The listing builds one solid part. Answer for the finished solid, in the listing's coordinates (mm). Face numbers are marked on the shaded views. A direction names the side the tool comes from. Give positions to 0.01 mm unless a question says otherwise; leave off trailing zeros. Order: outer loops, then holes, each group sorted by start corner. A loop starts at its lowest first (then second) coordinate and runs counter-clockwise, first axis right, second up. Notation, with made-up numbers: (65.25, -4) - (91.25, -4) arc R21 cw to (91.25, 7) - close; hole circle Ø8 at (-22, -11). An arc over 180 degrees is marked (long way). Use a Markdown table: item, result. Add a question column.
1) Find section A-A, the plane x = 90. Determine the outline of the cut face in (y, z).
2) For the marked faces 1 and 2, determine the directions among +Z, -Z, +X, -X, +Y, -Y from which every point of the face is accessible in a straight line to the end or side of a thin tool.
3) Straight lines are drawn through the part: line 1 (Y direction, x = -90, z = -52.4); line 2 (Z direction, x = -64, y = 19); line 3 (Y direction, x = -13, z = 21.5). For each, find the intervals that lie inside material, in ascending order.
4) Find section B-B, the plane y = 20. Determine the outline of the cut face in (x, z).
5) Flat-ended cylindrical pins translate along their axes: pin 1 (12 mm diameter, centred on x = 28, z = -39, fed in from +Y); pin 2 (12.5 mm diameter, centred on x = 2.5, y = 19, fed in from +Z). Find the tip coordinate at first contact, or state that the pin passes through.
6) Find section C-C, the plane z = 4. Determine the outline of the cut face in (x, y), plus the area to 3 significant figures.
7) Find section D-D, the plane x = -72. Determine the outline of the cut face in (y, z), plus the area to 3 significant figures.
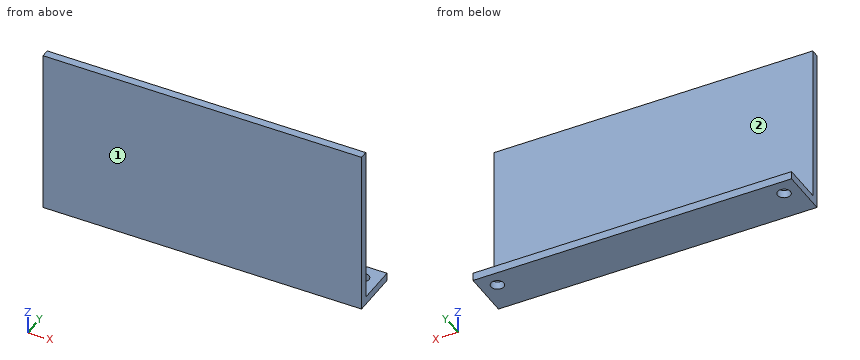
from build123d import *

# Parameters (mm, degrees)
SKETCH1_W           = 200
SKETCH1_H           = 100
BOSS_EXTRUDE1_DEPTH = 5
SKETCH2_W           = 200
SKETCH2_H           = 5
BOSS_EXTRUDE2_DEPTH = 30
SKETCH3_R           = 4
CUT_EXTRUDE1_DEPTH  = 40


with BuildPart() as part:
    # Sketch1 → Boss-Extrude1 (new body)
    with BuildSketch(Plane(origin=(0, 0, 0), x_dir=(1, 0, 0), z_dir=(0, 1, 0))):
        Rectangle(SKETCH1_W, SKETCH1_H)
    extrude(amount=BOSS_EXTRUDE1_DEPTH)

    # Sketch2 → Boss-Extrude2 (add)
    with BuildSketch(Plane.XZ):
        with Locations((0, -52.5)):
            Rectangle(SKETCH2_W, SKETCH2_H)
    extrude(amount=-BOSS_EXTRUDE2_DEPTH)

    # Sketch3 → Cut-Extrude1 (cut)
    with BuildSketch(Plane.XY.offset(-50)):
        with Locations((-90, 20)):
            Circle(SKETCH3_R)
        with Locations((90, 20)):
            Circle(SKETCH3_R)
    extrude(amount=-CUT_EXTRUDE1_DEPTH, mode=Mode.SUBTRACT)


solid = part.part
The answers:
| question | item | result |
|---|---|---|
| 1 | outline | (0, -55) - (16, -55) - (16, -50) - (5, -50) - (5, 50) - (0, 50) - close; (24, -55) - (30, -55) - (30, -50) - (24, -50) - close |
| 2 | face 1 | +Z, -Z, +X, -X, -Y |
| 2 | face 2 | +Z, +X, -X, +Y |
| 3 | line 1 | 0 to 16, 24 to 30 |
| 3 | line 2 | -55 to -50 |
| 3 | line 3 | 0 to 5 |
| 4 | outline | (-100, -55) - (-94, -55) - (-94, -50) - (-100, -50) - close; (-86, -55) - (86, -55) - (86, -50) - (-86, -50) - close; (94, -55) - (100, -55) - (100, -50) - (94, -50) - close |
| 5 | pin 1 | y = 5 |
| 5 | pin 2 | z = -50 |
| 6 | outline | (-100, 0) - (100, 0) - (100, 5) - (-100, 5) - close |
| 6 | area | 1,000 mm2 |
| 7 | outline | (0, -55) - (30, -55) - (30, -50) - (5, -50) - (5, 50) - (0, 50) - close |
| 7 | area | 650 mm2 |
